For this review, take the finished solid that the model builds, in its own axes (mm). A direction names the side the tool comes from. Round coordinates to 2 decimals unless told otherwise and drop trailing zeros. Write each loop counter-clockwise with the first axis right and the second up, starting at its lowest first coordinate (ties: lowest second). Pieces come first, ordered by that corner, then holes. Notation, with made-up numbers: M 76,-38 L 112,-38 A22 ccw 112,-27 Z; hole C 34.5,-20.75 d9. An arc over 180 degrees is marked long. Answer in a Markdown table with one row per item.
```python
from build123d import *

# Parameters (mm, degrees)
SKETCH1_W           = 30
SKETCH1_H           = 30
SKETCH1_R           = 1.6
SKETCH1_W_2         = 81.01
SKETCH1_H_2         = 12
BOSS_EXTRUDE1_DEPTH = 6
SKETCH1_3_W         = 30
SKETCH1_3_H         = 30
SKETCH1_3_R         = 1.6
BOSS_EXTRUDE2_DEPTH = 22.33
CUT_EXTRUDE1_DEPTH  = 88.671255266
SKETCH3_R           = 2.55
CUT_EXTRUDE2_DEPTH  = 8
CUT_EXTRUDE3_DEPTH  = 4.5
SKETCH6_R           = 5
CUT_EXTRUDE5_DEPTH  = 8.6
SKETCH7_R           = 1.6
CUT_EXTRUDE6_DEPTH  = 112.183402538
SKETCH8_R           = 2.85
CUT_EXTRUDE7_DEPTH  = 18
BOSS_EXTRUDE3_START = 2.43
SKETCH9_R           = 3.4
SKETCH9_R_2         = 2.55
BOSS_EXTRUDE3_DEPTH = 2.43
CHAMFER1_SIZE       = 1.2
FILLET3_R           = 4
CHAMFER2_SIZE       = 0.8
SKETCH10_R          = 2.5
CUT_EXTRUDE8_DEPTH  = 3
CHAMFER3_SIZE       = 0.8
BOSS_EXTRUDE6_DEPTH = 14
CUT_EXTRUDE10_REACH = 116.661
SKETCH17_R          = 1.1
FILLET5_R           = 2


with BuildPart() as part:
    # Sketch1 → Boss-Extrude1 (new body)
    # profile 1 of 2: a face of its own
    with BuildSketch(Plane.XY):
        with Locations((10, 10)):
            Rectangle(SKETCH1_W, SKETCH1_H)
        with Locations((20, 0)):
            Circle(SKETCH1_R, mode=Mode.SUBTRACT)
        with Locations((20, 20)):
            Circle(SKETCH1_R, mode=Mode.SUBTRACT)
        with Locations((0, 20)):
            Circle(SKETCH1_R, mode=Mode.SUBTRACT)
        Circle(SKETCH1_R, mode=Mode.SUBTRACT)
    # profile 2 of 2: a face of its own
    with BuildSketch(Plane.XY):
        with Locations((65.505, 10)):
            Rectangle(SKETCH1_W_2, SKETCH1_H_2)
    extrude(amount=BOSS_EXTRUDE1_DEPTH)

    # Sketch1<3> → Boss-Extrude2 (add)
    with BuildSketch(Plane.XY):
        with Locations((10, 10)):
            Rectangle(SKETCH1_3_W, SKETCH1_3_H)
        with Locations((20, 0)):
            Circle(SKETCH1_3_R, mode=Mode.SUBTRACT)
        with Locations((20, 20)):
            Circle(SKETCH1_3_R, mode=Mode.SUBTRACT)
        with Locations((0, 20)):
            Circle(SKETCH1_3_R, mode=Mode.SUBTRACT)
        Circle(SKETCH1_3_R, mode=Mode.SUBTRACT)
    extrude(amount=BOSS_EXTRUDE2_DEPTH)

    # Sketch2 → Cut-Extrude1 (cut, through all)
    with BuildSketch(Plane(origin=(25, 0, 0), x_dir=(0, 0, -1), z_dir=(1, 0, 0))):
        with BuildLine():
            Line((-6.515, 16.079632043), (-9.09, 16.079632043))
            Line((-9.09, 16.079632043), (-10.173218492, 15.888631397))
            ThreePointArc((-10.173218492, 15.888631397), (-11.235427971, 14.554192061), (-12.689983513, 15.444857819))
            Line((-12.689983513, 15.444857819), (-13.725, 15.262356487))
            Line((-13.725, 15.262356487), (-13.725, 4.536907598))
            Line((-13.725, 4.536907598), (-12.689983513, 4.354406266))
            ThreePointArc((-12.689983513, 4.354406266), (-11.235427971, 5.245072025), (-10.173218492, 3.910632689))
            Line((-10.173218492, 3.910632689), (-9.09, 3.719632043))
            Line((-9.09, 3.719632043), (-6.515, 3.719632043))
            Line((-6.515, 3.719632043), (-6, 4.234632043))
            Line((-6, 4.234632043), (-6, 15.564632043))
            Line((-6, 15.564632043), (-6.515, 16.079632043))
        make_face()
    extrude(amount=-CUT_EXTRUDE1_DEPTH, mode=Mode.SUBTRACT)

    # Sketch3 → Cut-Extrude2 (cut)
    with BuildSketch(Plane.XY.offset(22.33)):
        with Locations((10, 10)):
            Circle(SKETCH3_R)
    extrude(amount=-CUT_EXTRUDE2_DEPTH, mode=Mode.SUBTRACT)

    # Sketch5 → Cut-Extrude3 (cut)
    with BuildSketch(Plane(origin=(0, 0, 13.725), x_dir=(-1, 0, 0), z_dir=(0, 0, -1))):
        Polygon((-5.32346282, 10), (-7.66173141, 14.05), (-12.33826859, 14.05), (-14.67653718, 10), (-12.33826859, 5.95), (-7.66173141, 5.95), align=None)
    extrude(amount=-CUT_EXTRUDE3_DEPTH, mode=Mode.SUBTRACT)

    # Sketch6 → Cut-Extrude5 (cut)
    with BuildSketch(Plane(origin=(0, 0, 0), x_dir=(-1, 0, 0), z_dir=(0, 0, -1))):
        with Locations((-10, 10)):
            Circle(SKETCH6_R)
    extrude(amount=-CUT_EXTRUDE5_DEPTH, mode=Mode.SUBTRACT)

    # Sketch7 → Cut-Extrude6 (cut, through all)
    with BuildSketch(Plane(origin=(0, 0, 0), x_dir=(-1, 0, 0), z_dir=(0, 0, -1))):
        with BuildLine():
            ThreePointArc((-101.1, 10), (-99.5, 8.4), (-97.9, 10))
            Line((-97.9, 10), (-101.1, 10))
        make_face()
        with BuildLine():
            Line((-101.1, 10), (-97.9, 10))
            ThreePointArc((-97.9, 10), (-99.5, 11.6), (-101.1, 10))
        make_face()
        with Locations((-74.5, 10)):
            Circle(SKETCH7_R)
        with Locations((-49.5, 10)):
            Circle(SKETCH7_R)
    extrude(amount=-CUT_EXTRUDE6_DEPTH, mode=Mode.SUBTRACT)

    # Sketch8 → Cut-Extrude7 (cut)
    with BuildSketch(Plane.XY.offset(22.33)):
        with Locations((20, 20)):
            Circle(SKETCH8_R)
        with Locations((20, 0)):
            Circle(SKETCH8_R)
        Circle(SKETCH8_R)
        with Locations((0, 20)):
            Circle(SKETCH8_R)
    extrude(amount=-CUT_EXTRUDE7_DEPTH, mode=Mode.SUBTRACT)

    # Sketch9 → Boss-Extrude3 (add)
    with BuildSketch(Plane.XY.offset(22.33).offset(BOSS_EXTRUDE3_START)):
        with Locations(Location((10, 10, 0), (0, 0, 180))):
            Circle(SKETCH9_R)
        with Locations((10, 10)):
            Circle(SKETCH9_R_2, mode=Mode.SUBTRACT)
    extrude(amount=-BOSS_EXTRUDE3_DEPTH)

    # Chamfer1
    chamfer1_edges = [part.edges().sort_by_distance(p)[0] for p in [
        (13.4, 10, 22.33),
    ]]
    chamfer(chamfer1_edges, length=CHAMFER1_SIZE)

    # Fillet3
    fillet3_edges = [part.edges().sort_by_distance(p)[0] for p in [
        (-5, -5, 11.165),
        (-5, 25, 11.165),
        (25, 25, 11.165),
        (25, 16, 3),
        (106.01, 16, 3),
        (106.01, 4, 3),
        (25, 4, 3),
        (25, -5, 11.165),
    ]]
    fillet(fillet3_edges, radius=FILLET3_R)

    # Chamfer2
    chamfer2_edges = [part.edges().sort_by_distance(p)[0] for p in [
        (-2.85, 20, 22.33),
        (-2.85, 0, 22.33),
        (17.15, 0, 22.33),
        (17.15, 20, 22.33),
    ]]
    chamfer(chamfer2_edges, length=CHAMFER2_SIZE)

    # Sketch10 → Cut-Extrude8 (cut)
    with BuildSketch(Plane(origin=(0, 0, 0), x_dir=(-1, 0, 0), z_dir=(0, 0, -1))):
        with Locations((-99.5, 10)):
            Circle(SKETCH10_R)
        with Locations((-74.5, 10)):
            Circle(SKETCH10_R)
        with Locations((-49.5, 10)):
            Circle(SKETCH10_R)
    extrude(amount=-CUT_EXTRUDE8_DEPTH, mode=Mode.SUBTRACT)

    # Chamfer3
    chamfer3_edges = [part.edges().sort_by_distance(p)[0] for p in [
        (102, 10, 0),
        (77, 10, 0),
        (52, 10, 0),
    ]]
    chamfer(chamfer3_edges, length=CHAMFER3_SIZE)

    # Sketch15 → Boss-Extrude6 (add)
    with BuildSketch(Plane.XY.offset(22.33)):
        Polygon((18.343145751, 31), (12.343145751, 25), (18, 25), (21, 28), (27, 28), (27, 31), align=None)
    extrude(amount=-BOSS_EXTRUDE6_DEPTH)

    # Sketch17 → Cut-Extrude10 (cut, up to next)
    with BuildSketch(Plane(origin=(0, 31, 0), x_dir=(1, 0, 0), z_dir=(0, 1, 0)), mode=Mode.PRIVATE) as cut_extrude10_sk1:
        with Locations(Location((24, -11.33, 0), (0, 0, 180))):
            Circle(SKETCH17_R)
    cut_extrude10_tool1 = extrude(cut_extrude10_sk1.sketch, amount=-CUT_EXTRUDE10_REACH, mode=Mode.PRIVATE) & part.part
    # Sketch17 → Cut-Extrude10 (cut, up to next)
    with BuildSketch(Plane(origin=(0, 31, 0), x_dir=(1, 0, 0), z_dir=(0, 1, 0)), mode=Mode.PRIVATE) as cut_extrude10_sk2:
        with Locations(Location((24, -17.83, 0), (0, 0, 180))):
            Circle(SKETCH17_R)
    cut_extrude10_tool2 = extrude(cut_extrude10_sk2.sketch, amount=-CUT_EXTRUDE10_REACH, mode=Mode.PRIVATE) & part.part
    add(cut_extrude10_tool1.solids().sort_by_distance((24, 31, 11.33))[0], mode=Mode.SUBTRACT)
    add(cut_extrude10_tool2.solids().sort_by_distance((24, 31, 17.83))[0], mode=Mode.SUBTRACT)

    # Fillet5
    # the kernel refuses this fillet: 2 mm, written as the material it adds along each edge
    with BuildSketch(Plane(origin=(21, 28, 22.33), x_dir=(-0.7071067811865475, -0.7071067811865475, 0), z_dir=(0, 0, -1))) as fillet5_piece_1:
        with BuildLine():
            CenterArc((FILLET5_R * 0.414213562373, -FILLET5_R), FILLET5_R, 90, 45)
            Line((-FILLET5_R * 0.292893218813, -FILLET5_R * 0.292893218813), (0, 0))
            Line((0, 0), (FILLET5_R * 0.414213562373, 0))
        make_face()
    extrude(amount=14)
    with BuildSketch(Plane(origin=(12.343145751, 25, 22.33), x_dir=(-1, 0, 0), z_dir=(0, 0, -1))) as fillet5_piece_2:
        with BuildLine():
            CenterArc((FILLET5_R * 0.414213562373, FILLET5_R), FILLET5_R, 225, 45)
            Line((-FILLET5_R * 0.292893218813, FILLET5_R * 0.292893218813), (0, 0))
            Line((0, 0), (FILLET5_R * 0.414213562373, 0))
        make_face()
    extrude(amount=14)
    with BuildSketch(Plane(origin=(18, 25, 22.33), x_dir=(0.9993539414176275, -0.03594022500003582, 0), z_dir=(0, 0, -1))) as fillet5_piece_3:
        with BuildLine():
            CenterArc((4.541773641, -1.944797545), FILLET5_R, 103.492916805, 119.447416414)
            Line((3.07764659, -3.307270289), (2.931233885, -3.443517564))
            Line((2.931233885, -3.443517564), (-0.146412705, -0.136247274))
            Line((-0.146412705, -0.136247274), (0.007188045, 0.199870788))
            ThreePointArc((0.007188045, 0.199870788), (3.005249869, 0.092050113), (4.028458305, 0.194479755))
            Line((4.028458305, 0.194479755), (4.075123335, 0))
        make_face()
    extrude(amount=14)
    # the kernel refuses this fillet: 2 mm, written as the material it takes off along each edge
    with BuildSketch(Plane(origin=(27, 23, 22.33), x_dir=(-1, 0, 0), z_dir=(0, 1, 0))) as fillet5_2_piece_1:
        with BuildLine():
            CenterArc((FILLET5_R, -FILLET5_R), FILLET5_R, 90, 90)
            Line((0, -FILLET5_R), (0, 0))
            Line((0, 0), (FILLET5_R, 0))
        make_face()
    extrude(amount=13, mode=Mode.SUBTRACT)
    with BuildSketch(Plane(origin=(27, 23, 8.33), x_dir=(-1, 0, 0), z_dir=(0, 1, 0))) as fillet5_2_piece_2:
        with BuildLine():
            CenterArc((FILLET5_R, FILLET5_R), FILLET5_R, 180, 90)
            Line((0, FILLET5_R), (0, 0))
            Line((0, 0), (FILLET5_R, 0))
        make_face()
    extrude(amount=13, mode=Mode.SUBTRACT)
    with BuildSketch(Plane(origin=(18.343145751, 31, 24.401067812), x_dir=(-0.7071067811865476, -0.7071067811865476, 0), z_dir=(0, 0, -1))) as fillet5_2_piece_3:
        with BuildLine():
            CenterArc((FILLET5_R * 0.414213562373, -FILLET5_R), FILLET5_R, 90, 45)
            Line((-FILLET5_R * 0.292893218813, -FILLET5_R * 0.292893218813), (0, 0))
            Line((0, 0), (FILLET5_R * 0.414213562373, 0))
        make_face()
    extrude(amount=18.142135624, mode=Mode.SUBTRACT)


solid = part.part
```
Q1. Machinability: for faces 4 (the face through (10, 16.08, 8)), 5 (the face through (0, 18, 4.33)), 6 (the face through (13.491, 12.053, 15.944)), which of the approach directions +Z, -Z, +X, -X, +Y, -Y give a long, thin tool a straight path to every point of the face, cutting with its end or side? Answer none if there is none.
Found:
| item | result |
|---|---|
| face 4 | +X, -X |
| face 5 | +Z |
| face 6 | -Z |
Q2. Mouldability with a two-part tool opening along Y and no side actions: class faces 1 (the face through (104.807, 14.859, 3.042)), 2 (the face through (26.4, 29.5, 8.9)), 3 (the face through (47.19, 9.04, 1.88)) as +Y half, -Y half, draft (parallel to the pull), parting line (faces both ways), or undercut.
Found:
| item | result |
|---|---|
| face 1 | +Y half |
| face 2 | draft |
| face 3 | undercut |
Q3. For probe 1 along Y at (x, z) = (0, 16.75); probe 2 along Y at (x, z) = (20, 3.35), list the stretches that pass through material, from the lowest coordinate up.
Found:
| item | result |
|---|---|
| probe 1 | -5 to -2.85, 2.85 to 17.15, 22.85 to 25 |
| probe 2 | -5 to -1.6, 1.6 to 18.4, 21.6 to 25 |
Q4. Insertion check: P1, Ø3.5, axis at x = 20, y = 0, coming from the +Z side; P2, Ø6.5, axis at x = 11, y = 9, coming from the -Z side (3 decimals); P3, Ø5, axis at y = 26.5, z = 8, coming from the +X side; P4, Ø10, axis at y = 11, z = 9.5, coming from the +X side. Each pin has a flat end and moves straight along its axis. Give the tip position at first contact, or say it passes through.
Found:
| item | result |
|---|---|
| P1 | z = 4.33 |
| P2 | z = 13.725 |
| P3 | x = 26.97 |
| P4 | x = 106.01 |
Q5. Take a section at B-B (x = 74.5). State the section outline as (y, z) points.
Found:
| item | result |
|---|---|
| outline | M 4,0 L 6.7,0 L 7.5,0.8 L 7.5,3 L 8.4,3 L 8.4,6 L 4,6 Z; M 11.6,3 L 12.5,3 L 12.5,0.8 L 13.3,0 L 16,0 L 16,6 L 11.6,6 Z |
